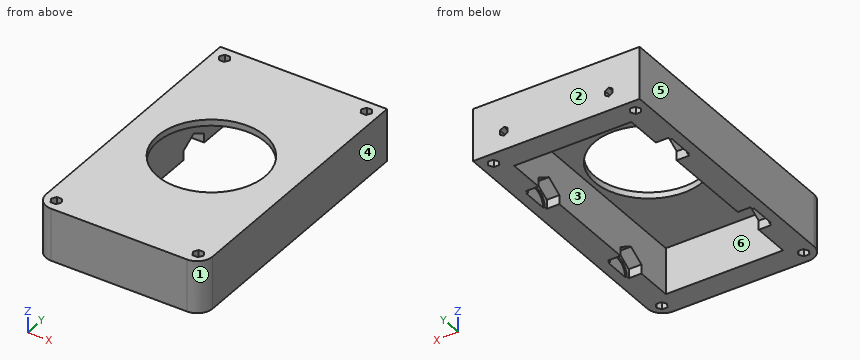
from build123d import *

# Parameters (mm, degrees)
SKETCH1_W           = 54
SKETCH1_H           = 90
SKETCH1_W_2         = 38
SKETCH1_H_2         = 74
BOSS_EXTRUDE1_DEPTH = 30
CUT_EXTRUDE1_DEPTH  = 4.1
SKETCH5_R           = 4.1
CUT_EXTRUDE2_DEPTH  = 0.5
CUT_EXTRUDE3_DEPTH  = 4.1
SKETCH7_R           = 4.1
CUT_EXTRUDE4_DEPTH  = 0.5
SKETCH8_W           = 54
SKETCH8_H           = 90
BOSS_EXTRUDE2_DEPTH = 2
SKETCH9_W           = 54
SKETCH9_H           = 90
BOSS_EXTRUDE3_DEPTH = 2
SKETCH12_W          = 54
SKETCH12_H          = 90
CUT_EXTRUDE7_DEPTH  = 17
CUT_EXTRUDE8_DEPTH  = 18
SKETCH14_R          = 17.5
CUT_EXTRUDE9_DEPTH  = 3
CUT_EXTRUDE10_DEPTH = 5
FILLET1_R           = 5


with BuildPart() as part:
    # Sketch1 → Boss-Extrude1 (new body)
    with BuildSketch(Plane.XY):
        with Locations((27, 45)):
            Rectangle(SKETCH1_W, SKETCH1_H)
        with Locations((27, 45)):
            Rectangle(SKETCH1_W_2, SKETCH1_H_2, mode=Mode.SUBTRACT)
    extrude(amount=BOSS_EXTRUDE1_DEPTH)

    # Sketch2 → Cut-Extrude1 (cut)
    with BuildSketch(Plane.ZY.offset(-46)):
        Polygon((20.888972746, 65), (17.944486373, 70.1), (12.055513627, 70.1), (9.111027254, 65), (12.055513627, 59.9), (17.944486373, 59.9), align=None)
        Polygon((20.888972746, 25), (17.944486373, 30.1), (12.055513627, 30.1), (9.111027254, 25), (12.055513627, 19.9), (17.944486373, 19.9), align=None)
    extrude(amount=-CUT_EXTRUDE1_DEPTH, mode=Mode.SUBTRACT)

    # Sketch5 → Cut-Extrude2 (cut)
    with BuildSketch(Plane.ZY.offset(-50.1)):
        with Locations((15, 65)):
            Circle(SKETCH5_R)
        with Locations((15, 25)):
            Circle(SKETCH5_R)
    extrude(amount=-CUT_EXTRUDE2_DEPTH, mode=Mode.SUBTRACT)

    # Sketch6 → Cut-Extrude3 (cut)
    with BuildSketch(Plane(origin=(8, 0, 0), x_dir=(0, 0, -1), z_dir=(1, 0, 0))):
        Polygon((-9.111027254, 65), (-12.055513627, 70.1), (-17.944486373, 70.1), (-20.888972746, 65), (-17.944486373, 59.9), (-12.055513627, 59.9), align=None)
        Polygon((-9.111027254, 25), (-12.055513627, 30.1), (-17.944486373, 30.1), (-20.888972746, 25), (-17.944486373, 19.9), (-12.055513627, 19.9), align=None)
    extrude(amount=-CUT_EXTRUDE3_DEPTH, mode=Mode.SUBTRACT)

    # Sketch7 → Cut-Extrude4 (cut)
    with BuildSketch(Plane(origin=(3.9, 0, 0), x_dir=(0, 0, -1), z_dir=(1, 0, 0))):
        with Locations((-15, 65)):
            Circle(SKETCH7_R)
        with Locations((-15, 25)):
            Circle(SKETCH7_R)
    extrude(amount=-CUT_EXTRUDE4_DEPTH, mode=Mode.SUBTRACT)

    # Sketch8 → Boss-Extrude2 (add)
    with BuildSketch(Plane.XY.offset(30)):
        with Locations((27, 45)):
            Rectangle(SKETCH8_W, SKETCH8_H)
    extrude(amount=BOSS_EXTRUDE2_DEPTH)

    # Sketch9 → Boss-Extrude3 (add)
    with BuildSketch(Plane(origin=(0, 0, 0), x_dir=(-1, 0, 0), z_dir=(0, 0, -1))):
        with Locations((-27, 45)):
            Rectangle(SKETCH9_W, SKETCH9_H)
    extrude(amount=BOSS_EXTRUDE3_DEPTH)

    # Sketch12 → Cut-Extrude7 (cut)
    with BuildSketch(Plane(origin=(0, 0, -2), x_dir=(-1, 0, 0), z_dir=(0, 0, -1))):
        with Locations((-27, 45)):
            Rectangle(SKETCH12_W, SKETCH12_H)
    extrude(amount=-CUT_EXTRUDE7_DEPTH, mode=Mode.SUBTRACT)

    # Sketch13 → Cut-Extrude8 (cut, through all)
    with BuildSketch(Plane(origin=(0, 0, 15), x_dir=(-1, 0, 0), z_dir=(0, 0, -1))):
        Polygon((-48.267949192, 86), (-49.133974596, 87.5), (-50.866025404, 87.5), (-51.732050808, 86), (-50.866025404, 84.5), (-49.133974596, 84.5), align=None)
        Polygon((-2.267949192, 86), (-3.133974596, 87.5), (-4.866025404, 87.5), (-5.732050808, 86), (-4.866025404, 84.5), (-3.133974596, 84.5), align=None)
        Polygon((-48.267949192, 4), (-49.133974596, 5.5), (-50.866025404, 5.5), (-51.732050808, 4), (-50.866025404, 2.5), (-49.133974596, 2.5), align=None)
        Polygon((-5.732050808, 4), (-4.866025404, 2.5), (-3.133974596, 2.5), (-2.267949192, 4), (-3.133974596, 5.5), (-4.866025404, 5.5), align=None)
    extrude(amount=-CUT_EXTRUDE8_DEPTH, mode=Mode.SUBTRACT)

    # Sketch14 → Cut-Extrude9 (cut, through all)
    with BuildSketch(Plane(origin=(0, 0, 30), x_dir=(-1, 0, 0), z_dir=(0, 0, -1))):
        with Locations((-27, 45)):
            Circle(SKETCH14_R)
    extrude(amount=-CUT_EXTRUDE9_DEPTH, mode=Mode.SUBTRACT)

    # Sketch15 → Cut-Extrude10 (cut)
    with BuildSketch(Plane(origin=(0, 90, 0), x_dir=(1, 0, 0), z_dir=(0, 1, 0))):
        Polygon((10, -19.556624327), (8.75, -20.278312164), (8.75, -21.721687836), (10, -22.443375673), (11.25, -21.721687836), (11.25, -20.278312164), align=None)
        Polygon((44, -19.556624327), (42.75, -20.278312164), (42.75, -21.721687836), (44, -22.443375673), (45.25, -21.721687836), (45.25, -20.278312164), align=None)
    extrude(amount=-CUT_EXTRUDE10_DEPTH, mode=Mode.SUBTRACT)

    # Fillet1
    fillet1_edges = [part.edges().sort_by_distance(p)[0] for p in [
        (54, 0, 23.5),
        (0, 0, 23.5),
    ]]
    fillet(fillet1_edges, radius=FILLET1_R)


solid = part.part
Verification items for the finished model (mm, model axes). Face numbers are marked on the shaded views. A direction names the side the tool comes from. Round coordinates to 2 decimals unless told otherwise and drop trailing zeros. Write each loop counter-clockwise with the first axis right and the second up, starting at its lowest first coordinate (ties: lowest second). Pieces come first, ordered by that corner, then holes.
(1) Material ranges on line 1 (X direction, y = 11.5, z = 22.75); line 2 (Y direction, x = 26, z = 28.5); line 3 (Y direction, x = 27, z = 31.2), recorded low to high.
Returned:
line 1: x = 0 to 8, 46 to 54
line 2: y = 0 to 8, 82 to 90
line 3: y = 0 to 27.5, 62.5 to 90
(2) Section check A-A (x = 27). Enter the section's corners in (y, z).
Returned:
outline: (0, 15) - (8, 15) - (8, 30) - (27.5, 30) - (27.5, 32) - (0, 32) - close; (62.5, 30) - (82, 30) - (82, 15) - (90, 15) - (90, 32) - (62.5, 32) - close
(3) Mould release check, pull along Y, two halves, no side actions. Record for the marked faces 1, 2, 3 and 4: pulls with the +Y half, pulls with the -Y half, needs draft (parallel to the pull), parting line crosses it, or undercut.
Returned:
face 1: pulls with the -Y half
face 2: pulls with the +Y half
face 3: undercut
face 4: needs draft
(4) Access from +Z, -Z, +X, -X, +Y, -Y to the whole of each face (thin tool, end or side, straight path). Record for the marked faces 5 and 6.
Returned:
face 5: +Z, -Z, -X, +Y, -Y
face 6: -Z
(5) Depth check by flat-ended pin: pin 1 Ø1.4 at (x, z) = (50, 24.5) entering from -Y; pin 2 Ø1 at (x, y) = (39.5, 24.5) entering from -Z; pin 3 Ø2 at (x, z) = (9.5, 21.5) entering from +Y. Enter the tip coordinate at first touch or a pass-through.
Returned:
pin 1: stops at y = 0.01
pin 2: stops at z = 30
pin 3: stops at y = 90
(6) Section check B-B (z = 27.25). Give the number of separate pieces and of enclosed holes in the cut face, plus the area to 3 significant figures.
Returned:
separate pieces: 1
enclosed holes: 5
area: 2,010 mm2
(7) Section check D-D (y = 9). Enter the section's corners in (x, z).
Returned:
outline: (0, 15) - (8, 15) - (8, 30) - (46, 30) - (46, 15) - (54, 15) - (54, 32) - (0, 32) - close
(8) Section check C-C (y = 45). Enter the section's corners in (x, z), plus the area to 3 significant figures.
Returned:
outline: (0, 15) - (8, 15) - (8, 30) - (9.5, 30) - (9.5, 32) - (0, 32) - close; (44.5, 30) - (46, 30) - (46, 15) - (54, 15) - (54, 32) - (44.5, 32) - close
area: 278 mm2
